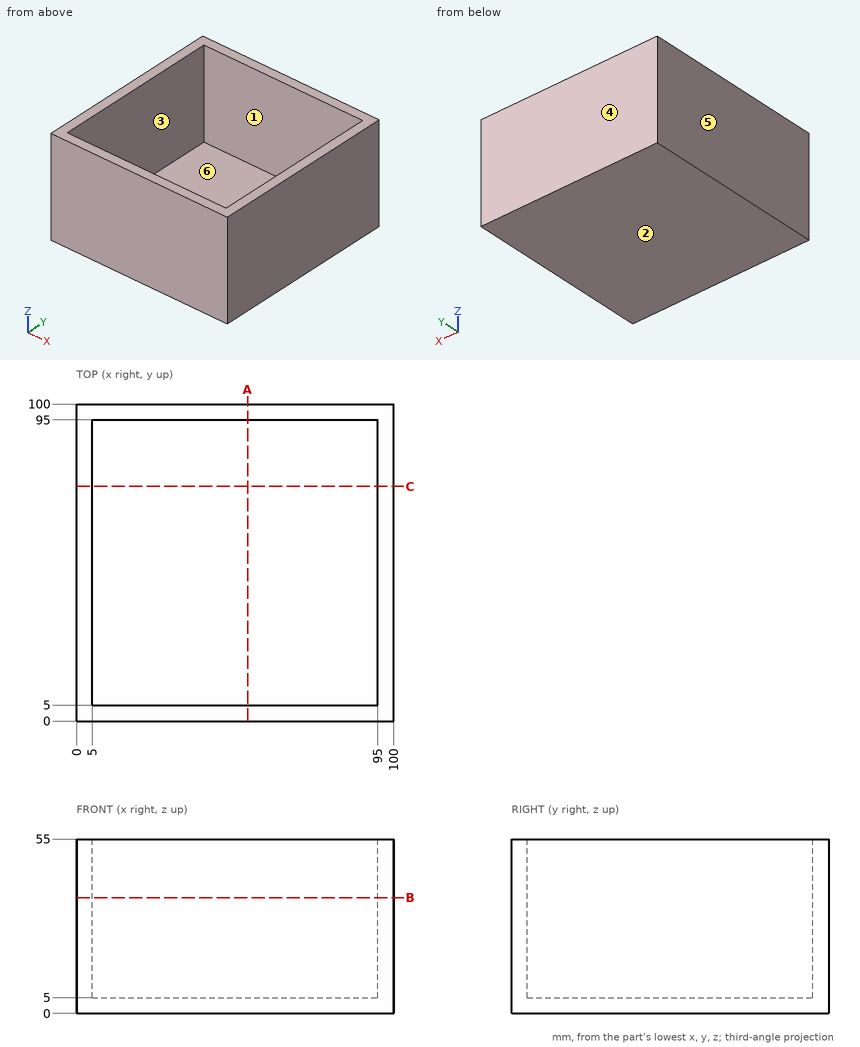
Geometry: see drawing. Coordinates: mm, zero at the bounding-box minimum. A direction names the side the tool comes from. Coordinates: 2 decimals unless noted, no trailing zeros. Write each loop counter-clockwise with the first axis right and the second up, starting at its lowest first coordinate (ties: lowest second). Pieces come first, ordered by that corner, then holes. Notation, with made-up numbers: M -20,-30 L -13,-30 A11 cw -13,-15 Z; hole C 18.25,12 d1. An arc over 180 degrees is marked long. Use CSV: the item, a comma, the result in double quotes. Start each with the question number.
1. Ray query, probe 1 along X at (y, z) = (9.5, 53.5); probe 2 along Z at (x, y) = (37, 29.5). Return the intervals inside material, ascending.
2. Mould query, pull axis Y, two halves, no side actions, for the marked faces 1, 2, 3 and 4. Classes: pulls with the +Y half, pulls with the -Y half, needs draft (parallel to the pull), parting line crosses it, or undercut.
3. Reachability of the marked faces 5 and 6 from +Z, -Z, +X, -X, +Y, -Y: full face, straight path, thin tool, end or side. Return the list, or none.
4. Cut plane B-B on z = 36.5. Return the cut outline in (x, y), plus the area to 3 significant figures.
5. Cut plane A-A on x = 54. Return the cut outline in (y, z).
6. First-contact query: P1, Ø6, axis at y = 81.5, z = 39, coming from the -X side; P2, Ø12, axis at x = 45.5, y = 20.5, coming from the +Z side. Flat tips, straight axial feed; report the tip coordinate or a pass-through.
Entries:
1,probe 1,"0 to 5, 95 to 100"
1,probe 2,"0 to 5"
2,face 1,"undercut"
2,face 2,"needs draft"
2,face 3,"undercut"
2,face 4,"pulls with the +Y half"
3,face 5,"+Z, -Z, -X, +Y, -Y"
3,face 6,"+Z"
4,outline,"M 0,0 L 100,0 L 100,100 L 0,100 Z; hole M 5,5 L 95,5 L 95,95 L 5,95 Z"
4,area,"1,900 mm²"
5,outline,"M 0,0 L 100,0 L 100,55 L 95,55 L 95,5 L 5,5 L 5,55 L 0,55 Z"
6,P1,"x = 0"
6,P2,"z = 5"
